Part model, mm, in its own coordinate system. A direction names the side the tool comes from. Give positions to 0.01 mm unless a question says otherwise; leave off trailing zeros. Order: outer loops, then holes, each group sorted by start corner. A loop starts at its lowest first (then second) coordinate and runs counter-clockwise, first axis right, second up. Notation, with made-up numbers: M 54.5,-27.75 L 102.5,-27.75 A13 cw 102.5,-15.75 Z; hole C -29.75,57.5 d11. An arc over 180 degrees is marked long. Return JSON: item names as keys, results as strings.
from build123d import *

# Parameters (mm, degrees)
SKETCH1_R           = 35
BOSS_EXTRUDE1_DEPTH = 100
SKETCH1_3_R         = 35
SKETCH1_3_R_2       = 30
CUT_EXTRUDE1_DEPTH  = 10
SKETCH1_4_R         = 27.5
CUT_EXTRUDE2_DEPTH  = 95
CHAMFER1_SIZE       = 1
FILLET1_R           = 1


with BuildPart() as part:
    # Sketch1 → Boss-Extrude1 (new body)
    with BuildSketch(Plane(origin=(0, 0, 0), x_dir=(1, 0, 0), z_dir=(0, 1, 0))):
        with Locations(Location((0, 0, 0), (0, 0, 270))):
            Circle(SKETCH1_R)
    extrude(amount=-BOSS_EXTRUDE1_DEPTH)

    # Sketch1_3 → Cut-Extrude1 (cut)
    with BuildSketch(Plane(origin=(0, 0, 0), x_dir=(1, 0, 0), z_dir=(0, 1, 0))):
        with Locations(Location((0, 0, 0), (0, 0, 270))):
            Circle(SKETCH1_3_R)
        with Locations(Location((0, 0, 0), (0, 0, 270))):
            Circle(SKETCH1_3_R_2, mode=Mode.SUBTRACT)
    extrude(amount=-CUT_EXTRUDE1_DEPTH, mode=Mode.SUBTRACT)

    # Sketch1_4 → Cut-Extrude2 (cut)
    with BuildSketch(Plane(origin=(0, 0, 0), x_dir=(1, 0, 0), z_dir=(0, 1, 0))):
        with Locations(Location((0, 0, 0), (0, 0, 270))):
            Circle(SKETCH1_4_R)
    extrude(amount=-CUT_EXTRUDE2_DEPTH, mode=Mode.SUBTRACT)

    # Chamfer1
    chamfer1_edges = [part.edges().sort_by_distance(p)[0] for p in [
        (0, -100, -35),
    ]]
    chamfer(chamfer1_edges, length=CHAMFER1_SIZE)

    # Fillet1
    fillet1_edges = [part.edges().sort_by_distance(p)[0] for p in [
        (0, 0, -27.5),
    ]]
    fillet(fillet1_edges, radius=FILLET1_R)


solid = part.part
Q1. Band-saw the part on B-B (z = 0). Give the cut face in (x, y), then the cut area to 3 significant figures.
Established:
{"outline": "M -35,-99 L -34,-100 L 34,-100 L 35,-99 L 35,-10 L 30,-10 L 30,0 L 28.5,0 A1 ccw 27.5,-1 L 27.5,-95 L -27.5,-95 L -27.5,-1 A1 ccw -28.5,0 L -30,0 L -30,-10 L -35,-10 Z", "area": "1,670 mm²"}
Q2. Probe line 1 along X through (y, z) = (-32.5, 1); line 2 along Y through (x, z) = (-32, -8); line 3 along Z through (x, y) = (2, -11.5). List the from-to ranges inside material, lowest first.
Established:
{"line 1": "x = -34.99 to -27.48, 27.48 to 34.99", "line 2": "y = -100 to -10", "line 3": "z = -34.94 to -27.43, 27.43 to 34.94"}
Q3. Pin check, flat tips, straight feed: pin 1 (2 mm diameter, centred on y = -69.5, z = -19, fed in from -X); pin 2 (4 mm diameter, centred on x = 14.5, z = -18, fed in from +Y); pin 3 (1 mm diameter, centred on y = -71.5, z = -19, fed in from +X). Stop position of each tip, or through.
Established:
{"pin 1": "stops at x = -30.02", "pin 2": "stops at y = -95", "pin 3": "stops at x = 29.71"}
Q4. Band-saw the part on A-A (y = -92.5). Give the cut face in (x, z).
Established:
{"outline": "C 0,0 d70; hole C 0,0 d55"}
Q5. Two-plate mould, pull along Z, no slides. Class faces 3 (the flat face through (16, -10, 26)), 4 (the flat face through (0, -95, 0)), 5 (the cylindrical face through (-21, -54, -28)): +Z half, -Z half, draft (parallel to the pull), parting line (faces both ways), or undercut.
Established:
{"face 3": "draft", "face 4": "undercut", "face 5": "parting line"}
Q6. 3-axis set-ups, long thin cutter, end or side, ignore diameter. For faces 1 (the cylindrical face through (1.32, -4.93, -29.97)), 2 (the flat face through (0, -100, 0)): which of +Z, -Z, +X, -X, +Y, -Y reach the whole face in a straight line?
Established:
{"face 1": "+Y", "face 2": "+Z, -Z, +X, -X, -Y"}
Q7. Band-saw the part on C-C (x = 0). Give the cut face in (y, z).
Established:
{"outline": "M -100,-34 L -99,-35 L -10,-35 L -10,-30 L 0,-30 L 0,-28.5 A1 ccw -1,-27.5 L -95,-27.5 L -95,27.5 L -1,27.5 A1 ccw 0,28.5 L 0,30 L -10,30 L -10,35 L -99,35 L -100,34 Z"}
